Here's how the part is built. I have some questions about the finished solid (model axes, mm). Coordinates: 2 decimals unless noted, no trailing zeros. Loops run counter-clockwise (first coordinate to the right, second up) from the corner with the lowest first, then second, coordinate; pieces in that order, holes last. Notation, with made-up numbers: (88.5, 81) - (125.5, 81) arc R12 cw to (125.5, 90) - close; hole circle Ø1 at (71, 57.5). An arc over 180 degrees is marked (long way). Use a Markdown table: item, result.
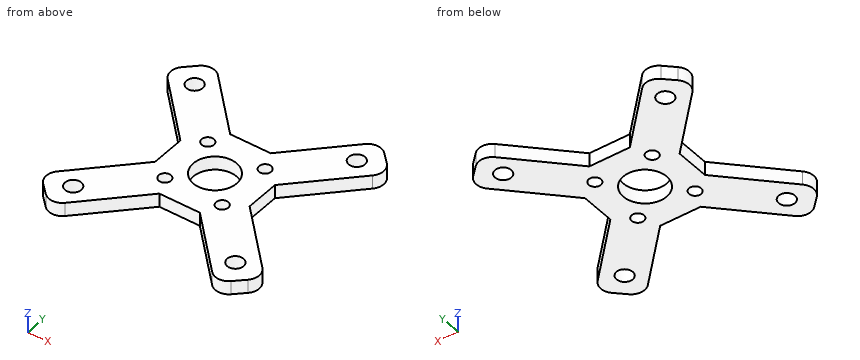
```python
from build123d import *

# Parameters (mm, degrees)
ESQUISSE1_R        = 8
ESQUISSE1_R_2      = 2.25
BOSS_EXTRU_1_DEPTH = 5
BOSS_EXTRU_2_START = -5
ESQUISSE2_R        = 3
BOSS_EXTRU_2_DEPTH = 5


with BuildPart() as part:
    # Esquisse1 → Boss.-Extru.1 (new body)
    with BuildSketch(Plane.XY):
        with BuildLine():
            Line((7.5, -17.5), (-7.5, -17.5))
            ThreePointArc((-7.5, -17.5), (-14.571067812, -14.571067812), (-17.5, -7.5))
            Line((-17.5, -7.5), (-17.5, 7.5))
            ThreePointArc((-17.5, 7.5), (-14.571067812, 14.571067812), (-7.5, 17.5))
            Line((-7.5, 17.5), (7.5, 17.5))
            ThreePointArc((7.5, 17.5), (14.571067812, 14.571067812), (17.5, 7.5))
            Line((17.5, 7.5), (17.5, -7.5))
            ThreePointArc((17.5, -7.5), (14.571067812, -14.571067812), (7.5, -17.5))
        make_face()
        Circle(ESQUISSE1_R, mode=Mode.SUBTRACT)
        with Locations((-10.605, 10.605)):
            Circle(ESQUISSE1_R_2, mode=Mode.SUBTRACT)
        with Locations((10.605, 10.605)):
            Circle(ESQUISSE1_R_2, mode=Mode.SUBTRACT)
        with Locations((-10.605, -10.605)):
            Circle(ESQUISSE1_R_2, mode=Mode.SUBTRACT)
        with Locations((10.605, -10.605)):
            Circle(ESQUISSE1_R_2, mode=Mode.SUBTRACT)
    extrude(amount=BOSS_EXTRU_1_DEPTH)

    # Esquisse2 → Boss.-Extru.2 (add)
    # profile 1 of 4: a face of its own
    with BuildSketch(Plane.XY.offset(5).offset(BOSS_EXTRU_2_START)):
        with BuildLine():
            Line((-37.944507823, 27.247644267), (-17.5, 6.269167951))
            Line((-17.5, 6.269167951), (-17.5, 7.5))
            ThreePointArc((-17.5, 7.5), (-14.571067812, 14.571067812), (-7.5, 17.5))
            Line((-7.5, 17.5), (-27.202072783, 37.7166504))
            ThreePointArc((-27.202072783, 37.7166504), (-30.718436651, 39.22656632), (-34.272553174, 37.807793369))
            Line((-34.272553174, 37.807793369), (-37.853364854, 34.318124658))
            ThreePointArc((-37.853364854, 34.318124658), (-39.363280773, 30.80176079), (-37.944507823, 27.247644267))
        make_face()
        with Locations((-30, 30)):
            Circle(ESQUISSE2_R, mode=Mode.SUBTRACT)
    # profile 2 of 4: a face of its own
    with BuildSketch(Plane.XY.offset(5).offset(BOSS_EXTRU_2_START)):
        with BuildLine():
            ThreePointArc((37.944507823, 27.247644267), (39.363280773, 30.80176079), (37.853364854, 34.318124658))
            Line((37.853364854, 34.318124658), (34.272553174, 37.807793369))
            ThreePointArc((34.272553174, 37.807793369), (30.718436651, 39.22656632), (27.202072783, 37.7166504))
            Line((27.202072783, 37.7166504), (7.5, 17.5))
            ThreePointArc((7.5, 17.5), (14.571067812, 14.571067812), (17.5, 7.5))
            Line((17.5, 7.5), (17.5, 6.269167951))
            Line((17.5, 6.269167951), (37.944507823, 27.247644267))
        make_face()
        with Locations((30, 30)):
            Circle(ESQUISSE2_R, mode=Mode.SUBTRACT)
    # profile 3 of 4: a face of its own
    with BuildSketch(Plane.XY.offset(5).offset(BOSS_EXTRU_2_START)):
        with BuildLine():
            Line((37.944507823, -27.247644267), (17.5, -6.269167951))
            Line((17.5, -6.269167951), (17.5, -7.5))
            ThreePointArc((17.5, -7.5), (14.571067812, -14.571067812), (7.5, -17.5))
            Line((7.5, -17.5), (27.202072783, -37.7166504))
            ThreePointArc((27.202072783, -37.7166504), (30.718436651, -39.22656632), (34.272553174, -37.807793369))
            Line((34.272553174, -37.807793369), (37.853364854, -34.318124658))
            ThreePointArc((37.853364854, -34.318124658), (39.363280773, -30.80176079), (37.944507823, -27.247644267))
        make_face()
        with Locations((30, -30)):
            Circle(ESQUISSE2_R, mode=Mode.SUBTRACT)
    # profile 4 of 4: a face of its own
    with BuildSketch(Plane.XY.offset(5).offset(BOSS_EXTRU_2_START)):
        with BuildLine():
            Line((-17.5, -7.5), (-17.5, -6.269167951))
            Line((-17.5, -6.269167951), (-37.944507823, -27.247644267))
            ThreePointArc((-37.944507823, -27.247644267), (-39.363280773, -30.80176079), (-37.853364854, -34.318124658))
            Line((-37.853364854, -34.318124658), (-34.272553174, -37.807793369))
            ThreePointArc((-34.272553174, -37.807793369), (-30.718436651, -39.22656632), (-27.202072783, -37.7166504))
            Line((-27.202072783, -37.7166504), (-7.5, -17.5))
            ThreePointArc((-7.5, -17.5), (-14.571067812, -14.571067812), (-17.5, -7.5))
        make_face()
        with Locations((-30, -30)):
            Circle(ESQUISSE2_R, mode=Mode.SUBTRACT)
    extrude(amount=BOSS_EXTRU_2_DEPTH)


solid = part.part
```
Q1. I want a section at A-A, the plane y = 0. Write out the boundary of the cut face in (x, z), then the cut area to 3 significant figures.
Check values:
| item | result |
|---|---|
| outline | (-17.5, 0) - (-8, 0) - (-8, 5) - (-17.5, 5) - close; (8, 0) - (17.5, 0) - (17.5, 5) - (8, 5) - close |
| area | 95.0 mm^2 |
Q2. I want a section at C-C, the plane z = 3.2. Give the number of separate pieces and of enclosed holes in the cut face, then the cut area to 3 significant figures.
Check values:
| item | result |
|---|---|
| separate pieces | 1 |
| enclosed holes | 9 |
| area | 2,610 mm^2 |
Q3. I want a section at D-D, the plane y = -30. Write out the boundary of the cut face in (x, z), then the cut area to 3 significant figures.
Check values:
| item | result |
|---|---|
| outline | (-39.31, 0) - (-33, 0) - (-33, 5) - (-39.31, 5) - close; (-27, 0) - (-19.68, 0) - (-19.68, 5) - (-27, 5) - close; (19.68, 0) - (27, 0) - (27, 5) - (19.68, 5) - close; (33, 0) - (39.31, 0) - (39.31, 5) - (33, 5) - close |
| area | 136 mm^2 |
Q4. Please list where these lines run through material, in increasing order: L1, parallel to Y at x = 10.5, z = 3.8; L2, parallel to Y at x = 30, z = 3.75; L3, parallel to X at y = -32.5, z = 1.75. Write a range as from..to.
Check values:
| item | result |
|---|---|
| L1 | -20.58..-12.85, -8.36..8.36, 12.85..20.58 |
| L2 | -39.17..-33, -27..-19.1, 19.1..27, 33..39.17 |
| L3 | -39.04..-31.66, -28.34..-22.12, 22.12..28.34, 31.66..39.04 |
Q5. Will these pins go through, and if not, where does the flat tip stop? P1, Ø1.5, axis at x = 9.5, z = 0.5, coming from the +Y side; P2, Ø4, axis at x = 10.605, y = -10.605, coming from the -Z side; P3, Ø2, axis at x = -25.5, z = 3.5, coming from the +Y side; P4, Ø1.5, axis at y = 2.5, z = 1.5, coming from the +X side.
Check values:
| item | result |
|---|---|
| P1 | y = 20.32 |
| P2 | through |
| P3 | y = 37 |
| P4 | x = 17.5 |
